The listing builds one solid part. Answer for the finished solid, in the listing's coordinates (mm). A direction names the side the tool comes from. Coordinates: 2 decimals unless noted, no trailing zeros. Order: outer loops, then holes, each group sorted by start corner. A loop starts at its lowest first (then second) coordinate and runs counter-clockwise, first axis right, second up. Notation, with made-up numbers: (5, 48.25) -> (31, 48.25) arc R19 cw to (31, 72.25) -> close; hole circle Ø1 at (1, -4). An arc over 180 degrees is marked (long way). One line per question, with ' | ' between items.
from build123d import *

# Parameters (mm, degrees)
F0_W      = 44
F0_H      = 77.1
F1_DEPTH  = 5
F2_W      = 27.6
F2_H      = 77.1
F3_DEPTH  = 5
F4_W      = 49
F4_H      = 27.6
F5_DEPTH  = 5
F6_W      = 49
F6_H      = 27.6
F7_DEPTH  = 5
F8_W      = 44
F8_H      = 3
F9_DEPTH  = 5
F10_W     = 3
F10_H     = 72.1
F11_DEPTH = 5
F12_W     = 39
F12_H     = 3
F13_DEPTH = 5
F14_W     = 44
F14_H     = 5
F15_DEPTH = 3
F16_R     = 2.5
F17_DEPTH = 12.7


with BuildPart() as f1:
    # F0 (on Front) → F1 (new body)
    with BuildSketch(Plane.XZ):
        with Locations((-0.431709, 22.922463)):
            Rectangle(F0_W, F0_H)
    extrude(amount=F1_DEPTH)

    # F2 (on face) → F3 (join)
    with BuildSketch(Plane(origin=(-22.431709, 0, 0), x_dir=(0, -1, 0), z_dir=(-1, 0, 0))):
        with Locations((13.8, 22.922463)):
            Rectangle(F2_W, F2_H)
    extrude(amount=F3_DEPTH)

    # F4 (on face) → F5 (join)
    with BuildSketch(Plane.XY.offset(61.472463)):
        with Locations((-2.931709, -13.8)):
            Rectangle(F4_W, F4_H)
    extrude(amount=F5_DEPTH)

    # F6 (on face) → F7 (join)
    with BuildSketch(Plane(origin=(0, 0, -15.627537), x_dir=(1, 0, 0), z_dir=(0, 0, -1))):
        with Locations((-2.931709, 13.8)):
            Rectangle(F6_W, F6_H)
    extrude(amount=F7_DEPTH)

    # F8 (on face) → F9 (join)
    with BuildSketch(Plane(origin=(0, 0, 61.472463), x_dir=(1, 0, 0), z_dir=(0, 0, -1))):
        with Locations((-0.431709, 21.5)):
            Rectangle(F8_W, F8_H)
    extrude(amount=F9_DEPTH)

    # F10 (on face) → F11 (join)
    with BuildSketch(Plane.YZ.offset(-22.431709)):
        with Locations((-21.5, 20.422463)):
            Rectangle(F10_W, F10_H)
    extrude(amount=F11_DEPTH)

    # F12 (on face) → F13 (join)
    with BuildSketch(Plane.XY.offset(-15.627537)):
        with Locations((2.068291, -21.5)):
            Rectangle(F12_W, F12_H)
    extrude(amount=F13_DEPTH)

    # F14 (on face) → F15 (join)
    with BuildSketch(Plane.XZ.offset(27.6)):
        Polygon((-27.431709, -20.627537), (21.568291, -20.627537), (21.568291, -15.627537), (-22.431709, -15.627537), (-27.431709, -15.627537), align=None)
        Polygon((-27.431709, 66.472463), (-27.431709, -15.627537), (-22.431709, -15.627537), (-22.431709, 61.472463), (-22.431709, 66.472463), align=None)
        with Locations((-0.431709, 63.972463)):
            Rectangle(F14_W, F14_H)
    extrude(amount=F15_DEPTH)

    # F16 (on face) → F17 (cut, symmetric)
    with BuildSketch(Plane.YZ.offset(-22.431709)):
        with Locations((-20, 22.922463)):
            Circle(F16_R)
    extrude(amount=F17_DEPTH, both=True, mode=Mode.SUBTRACT)


solid = f1.part
Item 1: Section B-B, the plane z = 42 is taken. Give the vertices of the cut face in (x, y), plus the area to 3 significant figures.
Computed values:
outline: (-27.43, -30.6) -> (-22.43, -30.6) -> (-22.43, -23) -> (-17.43, -23) -> (-17.43, -20) -> (-22.43, -20) -> (-22.43, -5) -> (21.57, -5) -> (21.57, 0) -> (-27.43, 0) -> close | area: 388 mm^2
Item 2: Determine the mould class of faces 1 (the face through (-1, -13, -15.628)), 2 (the face through (-1, -27, 61.472)), 3 (the face through (-1, -12, 61.472)), 4 (the face through (-3, 0, 24)) for opening direction Y: pulls with the +Y half, pulls with the -Y half, needs draft (parallel to the pull), parting line crosses it, or undercut.
Computed values:
face 1: undercut | face 2: needs draft | face 3: undercut | face 4: pulls with the +Y half
Item 3: Section A-A, the plane y = -21 is taken. Give the vertices of the cut face in (x, z), plus the area to 3 significant figures.
Computed values:
outline: (-27.43, -20.63) -> (21.57, -20.63) -> (21.57, -10.63) -> (-17.43, -10.63) -> (-17.43, 20.63) -> (-27.43, 20.63) -> close; (-27.43, 25.21) -> (-17.43, 25.21) -> (-17.43, 56.47) -> (21.57, 56.47) -> (21.57, 66.47) -> (-27.43, 66.47) -> close | area: 1,610 mm^2
Item 4: For faces 5 (the face through (-22.432, -27, 22)), 6 (the face through (-22.432, -12, 23)), 7 (the face through (21.568, -4, 19)), determine the directions among +Z, -Z, +X, -X, +Y, -Y from which every point of the face is accessible in a straight line to the end or side of a thin tool.
Computed values:
face 5: +X, -Y | face 6: +X | face 7: +Z, -Z, +X, +Y, -Y
Item 5: Section C-C, the plane x = 6 is taken. Give the vertices of the cut face in (y, z), plus the area to 4 significant figures.
Computed values:
outline: (-30.6, -20.63) -> (0, -20.63) -> (0, 66.47) -> (-30.6, 66.47) -> (-30.6, 61.47) -> (-23, 61.47) -> (-23, 56.47) -> (-20, 56.47) -> (-20, 61.47) -> (-5, 61.47) -> (-5, -15.63) -> (-20, -15.63) -> (-20, -10.63) -> (-23, -10.63) -> (-23, -15.63) -> (-30.6, -15.63) -> close | area: 721.5 mm^2
Item 6: Each of these flat-tipped pins is pushed along its axis until it touches: pin 1 Ø22 at (x, z) = (-8, 26) entering from -Y; pin 2 Ø1 at (y, z) = (-14.5, 18) entering from +X; pin 3 Ø1.5 at (y, z) = (-22, 22.5) entering from +X. Where does it stop, or does it pass through?
Computed values:
pin 1: stops at y = -23 | pin 2: stops at x = -22.43 | pin 3: stops at x = -17.43
Item 7: Find the intervals of material crossed by L1, parallel to Z at x = -23.25, y = -20; L2, parallel to Y at x = -22, z = -1; L3, parallel to Z at x = 15, y = -19.5, in increasing order.
Computed values:
L1: z = -20.63 to 20.42, 25.42 to 66.47 | L2: y = -23 to -20, -5 to 0 | L3: z = -20.63 to -15.63, 61.47 to 66.47
